```python
from build123d import *

# Parameters (mm, degrees)
SKETCH_1_R          = 16
EXTRUDE_1_DEPTH     = 9
SKETCH_2_R          = 6
EXTRUDE_2_DEPTH     = 0.5
SKETCH_3_R          = 16
EXTRUDE_3_DEPTH     = 3.25
SKETCH_4_R          = 5.5
EXTRUDE_4_DEPTH     = 2.25
SKETCH_5_R          = 3
CUT_EXTRUDE_1_DEPTH = 26.25
SKETCH_6_R          = 8
SKETCH_6_R_2        = 5.5
CUT_EXTRUDE_2_DEPTH = 2.25
SKETCH_7_R          = 0.6
CUT_EXTRUDE_3_DEPTH = 6
SKETCH_8_R          = 0.6
CUT_EXTRUDE_4_DEPTH = 3


with BuildPart() as part:
    # 草图1 → 凸台-拉伸1 (new body)
    with BuildSketch(Plane.XY):
        Circle(SKETCH_1_R)
    extrude(amount=EXTRUDE_1_DEPTH)

    # 草图2 → 凸台-拉伸2 (add)
    with BuildSketch(Plane.XY.offset(9)):
        Circle(SKETCH_2_R)
    extrude(amount=EXTRUDE_2_DEPTH)

    # 草图3 → 凸台-拉伸3 (add)
    with BuildSketch(Plane.XY.offset(9.5)):
        Circle(SKETCH_3_R)
    extrude(amount=EXTRUDE_3_DEPTH)

    # 草图4 → 凸台-拉伸4 (add)
    with BuildSketch(Plane.XY.offset(12.75)):
        Circle(SKETCH_4_R)
    extrude(amount=EXTRUDE_4_DEPTH)

    # 草图5 → 切除-拉伸1 (cut)
    with BuildSketch(Plane.XY.offset(15)):
        Circle(SKETCH_5_R)
    extrude(amount=-CUT_EXTRUDE_1_DEPTH, mode=Mode.SUBTRACT)

    # 草图6 → 切除-拉伸2 (cut)
    with BuildSketch(Plane.XY.offset(12.75)):
        Circle(SKETCH_6_R)
        Circle(SKETCH_6_R_2, mode=Mode.SUBTRACT)
    extrude(amount=-CUT_EXTRUDE_2_DEPTH, mode=Mode.SUBTRACT)

    # 草图7 → 切除-拉伸3 (cut)
    with BuildSketch(Plane(origin=(0, 0, 0), x_dir=(-1, 0, 0), z_dir=(0, 0, -1))):
        with Locations((8.660254038, 5)):
            Circle(SKETCH_7_R)
        with Locations((-8.660254038, 5)):
            Circle(SKETCH_7_R)
        with Locations((0, -10)):
            Circle(SKETCH_7_R)
    extrude(amount=-CUT_EXTRUDE_3_DEPTH, mode=Mode.SUBTRACT)

    # 草图8 → 切除-拉伸4 (cut)
    with BuildSketch(Plane.XY.offset(12.75)):
        with Locations((5, -8.660254038)):
            Circle(SKETCH_8_R)
        with Locations((5, 8.660254038)):
            Circle(SKETCH_8_R)
        with Locations((-10, 0)):
            Circle(SKETCH_8_R)
    extrude(amount=-CUT_EXTRUDE_4_DEPTH, mode=Mode.SUBTRACT)


solid = part.part
```
Here's how the part is built. I have some questions about the finished solid (model axes, mm). A direction names the side the tool comes from. Give positions to 0.01 mm unless a question says otherwise; leave off trailing zeros. Order: outer loops, then holes, each group sorted by start corner. A loop starts at its lowest first (then second) coordinate and runs counter-clockwise, first axis right, second up. Notation, with made-up numbers: (43.25, 16.5) -> (87.25, 16.5) arc R16 cw to (87.25, 34.5) -> close; hole circle Ø5 at (-38, 78.5). An arc over 180 degrees is marked (long way). Use CSV: the item, a comma, the result in double quotes. Start each with the question number.
Item 1: If I drill on probe 1 along Y at (x, z) = (0, 12); probe 2 along Z at (x, y) = (7, 4.5); probe 3 along Y at (x, z) = (5, 11.1) (3 decimals), over which ranges is the centre line in solid material (lowest first)? Write a range as [from, to].
Item 2: Suppose I cut it at C-C (z = 4). List the corners of the cut face in (x, y) for me.
Item 3: Thinking about a two-plate mould opening in Y: for faces 5 (the flat face through (7, 0, 9)), 6 (the flat face through (-10, 0, 9.75)), 7 (the cylindrical face through (-5.994, 0.264, 9.246)), which applies, pulls with the +Y half, pulls with the -Y half, needs draft (parallel to the pull), parting line crosses it, or undercut?
Item 4: Suppose I cut it at A-A (x = -10). List the corners of the cut face in (y, z) for me.
Item 5: Suppose I cut it at B-B (y = 6.5). List the corners of the cut face in (x, z) for me, and give its area (3 significant figures).
Item 6: On a 3-axis mill with a long thin cutter (end or side, diameter ignored), from which of +Z, -Z, +X, -X, +Y, -Y can I reach the whole of each face in a straight line? I mean faces 1 (the flat face through (7, 0, 9.5)), 2 (the flat face through (2.4, -2.4, 15)), 3 (the cylindrical face through (-1.19, -5.37, 12.78)), 4 (the flat face through (0, -10, 6)). Say none if no direction works.
Item 7: Suppose I cut it at D-D (x = -4). List the corners of the cut face in (y, z) for me, and give its area (3 significant figures).
Item 8: I'm going to push flat-ended pins straight in: P1, Ø0.6, axis at x = -10, y = 0, coming from the +Z side; P2, Ø0.6, axis at x = 5, y = 9, coming from the +Z side; P3, Ø8, axis at y = 6.5, z = 3, coming from the -X side. Where does each tip first touch, or does it pass through?
Answer block:
1,probe 1,"y = [-16, -8], [-5.5, -3], [3, 5.5], [8, 16]"
1,probe 2,"z = [0, 9], [9.5, 12.75]"
1,probe 3,"y = [-15.199, -9.26], [-8.06, -6.245], [-2.291, 2.291], [6.245, 8.06], [9.26, 15.199]"
2,outline,"circle Ø32 at (0, 0); hole circle Ø1.2 at (-8.66, 5); hole circle Ø6 at (0, 0); hole circle Ø1.2 at (0, -10); hole circle Ø1.2 at (8.66, 5)"
3,face 5,"needs draft"
3,face 6,"undercut"
3,face 7,"parting line crosses it"
4,outline,"(-12.49, 0) -> (12.49, 0) -> (12.49, 9) -> (-12.49, 9) -> close; (-12.49, 9.5) -> (12.49, 9.5) -> (12.49, 12.75) -> (0.6, 12.75) -> (0.6, 9.75) -> (-0.6, 9.75) -> (-0.6, 12.75) -> (-12.49, 12.75) -> close"
5,outline,"(-14.62, 0) -> (14.62, 0) -> (14.62, 9) -> (-14.62, 9) -> close; (-14.62, 9.5) -> (14.62, 9.5) -> (14.62, 12.75) -> (4.66, 12.75) -> (4.66, 10.5) -> (-4.66, 10.5) -> (-4.66, 12.75) -> (-14.62, 12.75) -> close"
5,area,"337 mm^2"
6,face 1,"none"
6,face 2,"+Z, +X, -X, +Y, -Y"
6,face 3,"+Z"
6,face 4,"-Z"
7,outline,"(-15.49, 0) -> (15.49, 0) -> (15.49, 9) -> (4.47, 9) -> (4.47, 9.5) -> (15.49, 9.5) -> (15.49, 12.75) -> (6.93, 12.75) -> (6.93, 10.5) -> (3.77, 10.5) -> (3.77, 15) -> (-3.77, 15) -> (-3.77, 10.5) -> (-6.93, 10.5) -> (-6.93, 12.75) -> (-15.49, 12.75) -> (-15.49, 9.5) -> (-4.47, 9.5) -> (-4.47, 9) -> (-15.49, 9) -> close"
7,area,"387 mm^2"
8,P1,"stops at z = 9.75"
8,P2,"stops at z = 12.75"
8,P3,"stops at x = -15.8"
